Read the model definition and answer for the solid it produces. Units are mm, in the model's axes. A direction names the side the tool comes from. Give positions to 0.01 mm unless a question says otherwise; leave off trailing zeros. Loops run counter-clockwise (first coordinate to the right, second up) from the corner with the lowest first, then second, coordinate; pieces in that order, holes last. Notation, with made-up numbers: (-4, 79.5) - (13, 79.5) arc R20 cw to (13, 117.5) - close; hole circle Ø2 at (31.5, 53.25). An arc over 180 degrees is marked (long way). Use a Markdown table: item, result. Add a question column.
Item 1: Which of the six approach directions +Z, -Z, +X, -X, +Y, -Y give full straight-line access (tool end or side, diameter ignored) to faces 4 (the face through (2.1, 10, 10.4)), 5 (the face through (-0.9, 17.5, 2.3)), 6 (the face through (-9.981, -0.14, 27.147))?
Item 2: A cutting plane is placed at A-A (z = 19.5). Determine the outline of the cut face in (x, y).
Item 3: A cutting plane is placed at B-B (y = -13.5). Determine the outline of the cut face in (x, z).
Item 4: For a pull along Y with two mould halves and no side action, classify faces 1 (the face through (0, -19, 5)), 2 (the face through (-12.5, 0, 5)), 3 (the face through (0, -14, 8)) as +Y half, -Y half, draft (parallel to the pull), parting line (faces both ways), or undercut.
Item 5: A cutting plane is placed at D-D (z = 11). Determine the outline of the cut face in (x, y), plus the area to 3 significant figures.
Item 6: Consider probe 1 along Y at (x, z) = (0, 2.2); probe 2 along X at (y, z) = (-3.25, 19.5); probe 3 along X at (y, z) = (-13.5, 2). Determine where each line is inside the solid, lowest interval first. Write a range as [from, to].
Item 7: A cutting plane is placed at C-C (x = 0). Determine the outline of the cut face in (y, z).
Item 8: Each of these flat-tipped pins is pushed along its axis until it touches: P1, Ø6.5, axis at x = 0, y = 13.5, coming from the +Z side; P2, Ø3, axis at y = 9, z = 7, coming from the +X side; P3, Ø0.5, axis at x = 0, y = -14, coming from the -Z side. Where does it stop, or does it pass through?
from build123d import *

# Parameters (mm, degrees)
SKETCH_W     = 25
SKETCH_H     = 38
PAD_DEPTH    = 10
SKETCH001_R  = 4.1
POCKET_DEPTH = 8
CHAMFER_SIZE = 3.3
PAD001_DEPTH = 10


with BuildPart() as part:
    # Sketch → Pad (new body)
    with BuildSketch(Plane.XY):
        Rectangle(SKETCH_W, SKETCH_H)
    extrude(amount=PAD_DEPTH)

    # Sketch001 (on Face5 of Pad) → Pocket (cut)
    with BuildSketch(Plane(origin=(0, 0, 0), x_dir=(1, 0, 0), z_dir=(0, 0, -1))):
        with Locations((0, 13.5)):
            Circle(SKETCH001_R)
        with Locations((0, -13.5)):
            Circle(SKETCH001_R)
    extrude(amount=-POCKET_DEPTH, mode=Mode.SUBTRACT)

    # Chamfer
    chamfer_edges = [part.edges().sort_by_distance(p)[0] for p in [
        (-4.1, 13.5, 8),
        (-4.1, -13.5, 8),
    ]]
    chamfer(chamfer_edges, length=CHAMFER_SIZE)

    # Sketch003 → Pad001 (join, symmetric)
    with BuildSketch(Plane.XZ):
        with BuildLine():
            ThreePointArc((-7, 25.156854), (0, 10.5), (7, 25.156854))
            ThreePointArc((8.619316, 27.987645), (6.842084, 27.125738), (7, 25.156854))
            Line((8.619316, 27.987645), (10.597427, 27.692553))
            Line((10.597427, 27.692553), (9.347427, 26.586053))
            Line((9.347427, 26.586053), (13.138853, 22.601698))
            ThreePointArc((6, 7.406613), (12.218698, 13.759493), (13.138853, 22.601698))
            Line((-6, 7.406613), (6, 7.406613))
            ThreePointArc((-13.138853, 22.601698), (-12.218698, 13.759493), (-6, 7.406613))
            Line((-9.347427, 26.586053), (-13.138853, 22.601698))
            Line((-10.597427, 27.692553), (-9.347427, 26.586053))
            Line((-8.619316, 27.987645), (-10.597427, 27.692553))
            ThreePointArc((-7, 25.156854), (-6.842084, 27.125738), (-8.619316, 27.987645))
        make_face()
    extrude(amount=PAD001_DEPTH, both=True)


solid = part.part
Geometry says:
| question | item | result |
|---|---|---|
| 1 | face 4 | +Z, +X, -X, +Y |
| 1 | face 5 | -Z |
| 1 | face 6 | -X, +Y, -Y |
| 2 | outline | (-13.5, -10) - (-9, -10) - (-9, 10) - (-13.5, 10) - close; (9, -10) - (13.5, -10) - (13.5, 10) - (9, 10) - close |
| 3 | outline | (-12.5, 0) - (-4.1, 0) - (-4.1, 4.7) - (-0.8, 8) - (0.8, 8) - (4.1, 4.7) - (4.1, 0) - (12.5, 0) - (12.5, 10) - (-12.5, 10) - close |
| 4 | face 1 | -Y half |
| 4 | face 2 | draft |
| 4 | face 3 | undercut |
| 5 | outline | (-10.49, -10) - (-2.96, -10) - (-2.96, 10) - (-10.49, 10) - close; (2.96, -10) - (10.49, -10) - (10.49, 10) - (2.96, 10) - close |
| 5 | area | 301 mm² |
| 6 | probe 1 | [-19, -17.6], [-9.4, 9.4], [17.6, 19] |
| 6 | probe 2 | [-13.5, -9], [9, 13.5] |
| 6 | probe 3 | [-12.5, -4.1], [4.1, 12.5] |
| 7 | outline | (-19, 0) - (-17.6, 0) - (-17.6, 4.7) - (-14.3, 8) - (-12.7, 8) - (-9.4, 4.7) - (-9.4, 0) - (9.4, 0) - (9.4, 4.7) - (12.7, 8) - (14.3, 8) - (17.6, 4.7) - (17.6, 0) - (19, 0) - (19, 10) - (10, 10) - (10, 10.5) - (-10, 10.5) - (-10, 10) - (-19, 10) - close |
| 8 | P1 | z = 10 |
| 8 | P2 | x = 12.5 |
| 8 | P3 | z = 8 |
